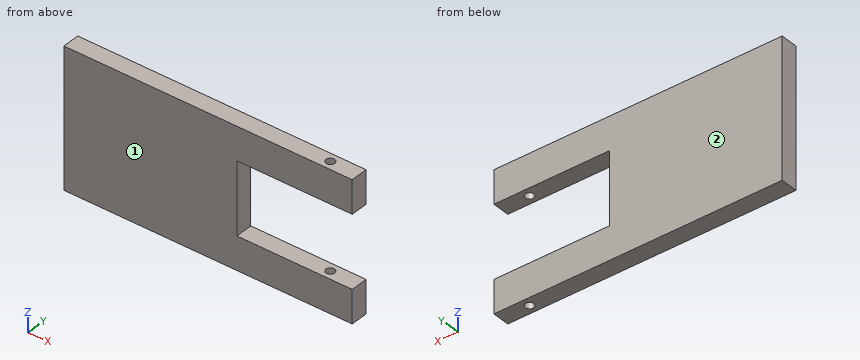
Autodesk Inventor part; units mm, degrees
ref_plane "YZ Plane" through (0, 0, 0) normal (1, 0, 0) x (0, 1, 0)
ref_plane "XZ Plane" through (0, 0, 0) normal (0, 1, 0) x (-1, 0, 0)
ref_plane "XY Plane" through (0, 0, 0) normal (0, 0, 1) x (1, 0, 0)
sketch "Sketch1" plane through (0, 0, 0) normal (0, 1, 0) x (-1, 0, 0)
  line L0 (-50, 24) -> (50, 24)
  line L1 (50, 24) -> (50, -24)
  line L2 (50, -24) -> (-50, -24)
  line L3 (-50, -24) -> (-50, 24)
  point P0 (0, 0)
  point P1 (-50, 0)
  point P2 (0, 24)
  point P3 (-5, -14)
  dimension "d0" = 100
  dimension "d1" = 48
  dimension "d4" = 45
  dimension "d5" = 10
extrude "Extrusion1" add sketch "Sketch1" against normal blind 6
sketch "Sketch2" plane through (0, 0, 0) normal (0, 1, 0) x (1, 0, 0)
  line L0 (50, 24) -> (-50, 24)
  line L1 (-50, 24) -> (-50, -24)
  line L2 (-50, -24) -> (50, -24)
  line L3 (50, -24) -> (50, 24)
  line L4 (50, 24) -> (50, -24)
  line L5 (50, -12.5) -> (10, -12.5)
  line L6 (10, -12.5) -> (10, 12.5)
  line L7 (10, 12.5) -> (50, 12.5)
  line L8 (50, 12.5) -> (50, -12.5)
  point P0 (0, 0)
  point P1 (10, 0)
  dimension "d6" = 40
  dimension "d7" = 25
extrude "Extrusion2" cut sketch "Sketch2" against normal blind 6 contours L3 L5 L6 L7
sketch "Sketch4" plane through (50, 0, -24) normal (0, 0, -1) x (-1, 0, 0)
  line L0 (0, 0) -> (0, -6)
  point P0 (50, 0)
  point P1 (10, -3)
  point P2 (0, -3)
  dimension "d12" = 10
hole "Hole1" at (40, -3, -24) direction (0, 0, 1) diameter 3 end through all
properties part number "Mausefallle" material "Wood (Oak)"
Design review of the part built by this model. Coordinates are the model's own, in mm. Face numbers are marked on the shaded views. Round coordinates to 2 decimals unless told otherwise and drop trailing zeros. Order: outer loops, then holes, each group sorted by start corner. A loop starts at its lowest first (then second) coordinate and runs counter-clockwise, first axis right, second up.
1) Clearance check with a flat-ended pin moving along its axis: pin 1 Ø1.8 at (y, z) = (-4.5, 2) entering from +X. State where the tip first meets the part, or that it passes through.
The answers:
pin 1: stops at x = 10
2) Consider section B-B (y = -3). State the section outline as (x, z) points.
The answers:
outline: (-50, -24) - (38.5, -24) - (38.5, -12.5) - (10, -12.5) - (10, 12.5) - (38.5, 12.5) - (38.5, 24) - (-50, 24) - close; (41.5, -24) - (50, -24) - (50, -12.5) - (41.5, -12.5) - close; (41.5, 12.5) - (50, 12.5) - (50, 24) - (41.5, 24) - close
3) Consider section A-A (x = 40). State the section outline as (y, z) points, plus the area to 3 significant figures.
The answers:
outline: (-6, -24) - (-4.5, -24) - (-4.5, -12.5) - (-6, -12.5) - close; (-6, 12.5) - (-4.5, 12.5) - (-4.5, 24) - (-6, 24) - close; (-1.5, -24) - (0, -24) - (0, -12.5) - (-1.5, -12.5) - close; (-1.5, 12.5) - (0, 12.5) - (0, 24) - (-1.5, 24) - close
area: 69.0 mm2
4) For L1, parallel to Y at x = 40, z = 20.5; L2, parallel to Z at x = 21.5, y = -3.05; L3, parallel to X at y = -3, z = 20.75, list the stretches that pass through material, from the lowest coordinate up.
The answers:
L1: y = -6 to -4.5, -1.5 to 0
L2: z = -24 to -12.5, 12.5 to 24
L3: x = -50 to 38.5, 41.5 to 50
5) Draft analysis for pull direction Y (two halves, no side actions). For the marked faces 1 and 2, state which applies: released by +Y, released by -Y, zero draft, split by the parting line, or undercut.
The answers:
face 1: released by -Y
face 2: released by +Y
6) Consider section C-C (x = 16). State the section outline as (y, z) points.
The answers:
outline: (-6, -24) - (0, -24) - (0, -12.5) - (-6, -12.5) - close; (-6, 12.5) - (0, 12.5) - (0, 24) - (-6, 24) - close
7) Consider section D-D (z = -4.5). State the section outline as (x, y) points, plus the area to 3 significant figures.
The answers:
outline: (-50, -6) - (10, -6) - (10, 0) - (-50, 0) - close
area: 360 mm2
